Input: dimensioned drawing with shaded views. Units: mm. Origin: part minimum x, y, z. Give positions to 0.01 mm unless a question says otherwise; leave off trailing zeros. Loops run counter-clockwise (first coordinate to the right, second up) from the corner with the lowest first, then second, coordinate; pieces in that order, holes last.
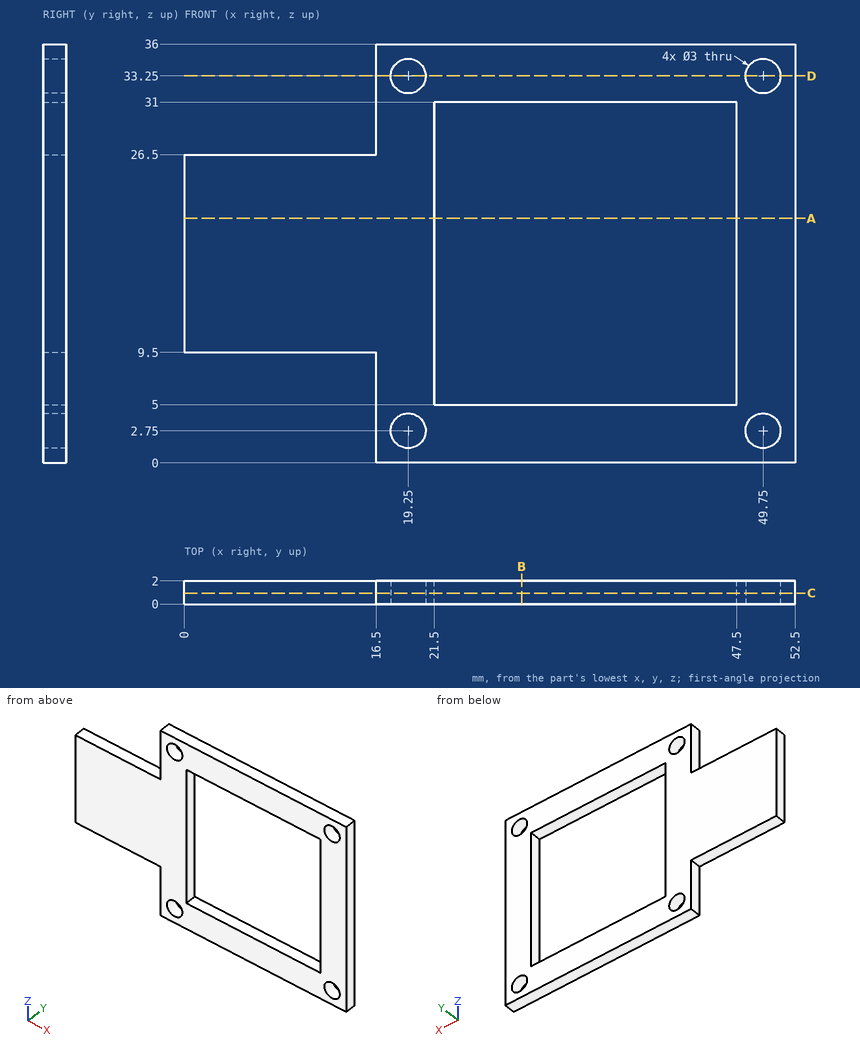
(1) Section D-D, the plane z = 33.25. Return the cut outline in (x, y), then the cut area to 3 significant figures.
A:
outline: (16.5, 0) - (17.75, 0) - (17.75, 2) - (16.5, 2) - close; (20.75, 0) - (48.25, 0) - (48.25, 2) - (20.75, 2) - close; (51.25, 0) - (52.5, 0) - (52.5, 2) - (51.25, 2) - close
area: 60.0 mm2
(2) Section A-A, the plane z = 21. Return the cut outline in (x, y).
A:
outline: (0, 0) - (21.5, 0) - (21.5, 2) - (0, 2) - close; (47.5, 0) - (52.5, 0) - (52.5, 2) - (47.5, 2) - close
(3) Section B-B, the plane x = 29. Return the cut outline in (y, z), then the cut area to 3 significant figures.
A:
outline: (0, 0) - (2, 0) - (2, 5) - (0, 5) - close; (0, 31) - (2, 31) - (2, 36) - (0, 36) - close
area: 20.0 mm2
(4) Section C-C, the plane y = 0.95. Return the cut outline in (x, z), then the cut area to 3 significant figures.
A:
outline: (0, 9.5) - (16.5, 9.5) - (16.5, 0) - (52.5, 0) - (52.5, 36) - (16.5, 36) - (16.5, 26.5) - (0, 26.5) - close; hole circle Ø3 at (19.25, 2.75); hole circle Ø3 at (19.25, 33.25); hole (21.5, 5) - (47.5, 5) - (47.5, 31) - (21.5, 31) - close; hole circle Ø3 at (49.75, 2.75); hole circle Ø3 at (49.75, 33.25)
area: 872 mm2
(5) First-contact query: pin 1 (1 mm diameter, centred on y = 1, z = 29.5, fed in from -X); pin 2 (0.6 mm diameter, centred on x = 7, y = 1, fed in from -Z); pin 3 (0.6 mm diameter, centred on x = 6.5, y = 1.5, fed in from +Z). Flat tips, straight axial feed; report the tip coordinate or a pass-through.
A:
pin 1: stops at x = 16.5
pin 2: stops at z = 9.5
pin 3: stops at z = 26.5
(6) Ray query, line 1 along X through (y, z) = (0.8, 2.75); line 2 along X through (y, z) = (0.5, 16); line 3 along Z through (x, y) = (46.5, 0.7). Return the intervals inside material, ascending.
A:
line 1: x = 16.5 to 17.75, 20.75 to 48.25, 51.25 to 52.5
line 2: x = 0 to 21.5, 47.5 to 52.5
line 3: z = 0 to 5, 31 to 36
